Verification items for the finished model (mm, model axes). Give positions to 0.01 mm unless a question says otherwise; leave off trailing zeros. Order: outer loops, then holes, each group sorted by start corner. A loop starts at its lowest first (then second) coordinate and runs counter-clockwise, first axis right, second up. Notation, with made-up numbers: (33.25, -28.75) - (89.25, -28.75) arc R36 ccw to (89.25, 6.25) - close; hole circle Ø3 at (17.5, 56.25). An arc over 180 degrees is marked (long way). Answer as a JSON object with one key per item and string values.
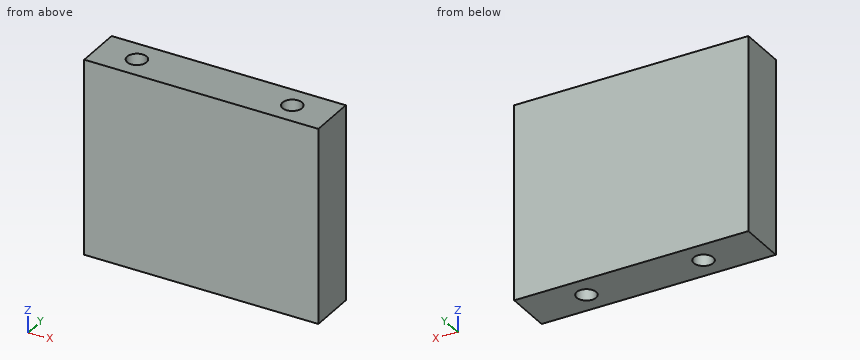
```python
from build123d import *

# Parameters (mm, degrees)
ESQUISSE1_W                                   = 30
ESQUISSE1_H                                   = 25
BOSS_EXTRU_1_DEPTH                            = 6
TROU_POUR_TARAUDAGE_POUR_TROU_TARAUD_M3_D     = 2.5
TROU_POUR_TARAUDAGE_POUR_TROU_TARAUD_M3_DEPTH = 10
TROU_POUR_TARAUDAGE_POUR_TROU_TARAUD_M3_TIP   = 0.751075774
TROU_POUR_TARAUDAGE_POUR_TROU_TARAUD_2_D      = 2.5
TROU_POUR_TARAUDAGE_POUR_TROU_TARAUD_2_DEPTH  = 11
TROU_POUR_TARAUDAGE_POUR_TROU_TARAUD_2_TIP    = 0.751075774


with BuildPart() as part:
    # Esquisse1 → Boss.-Extru.1 (new body)
    with BuildSketch(Plane(origin=(0, 0, 0), x_dir=(1, 0, 0), z_dir=(0, 1, 0))):
        Rectangle(ESQUISSE1_W, ESQUISSE1_H)
    extrude(amount=BOSS_EXTRU_1_DEPTH)

    # Trou pour taraudage pour trou taraud_ M3
    with Locations(Plane.XY.offset(12.5)):
        with Locations((-10, 3), (9.903892631, 3.003728502)):
            Hole(TROU_POUR_TARAUDAGE_POUR_TROU_TARAUD_M3_D / 2, depth=TROU_POUR_TARAUDAGE_POUR_TROU_TARAUD_M3_DEPTH)
            with Locations((0, 0, -(TROU_POUR_TARAUDAGE_POUR_TROU_TARAUD_M3_DEPTH + TROU_POUR_TARAUDAGE_POUR_TROU_TARAUD_M3_TIP / 2))):  # 118° drill point
                Cone(0, TROU_POUR_TARAUDAGE_POUR_TROU_TARAUD_M3_D / 2, TROU_POUR_TARAUDAGE_POUR_TROU_TARAUD_M3_TIP, mode=Mode.SUBTRACT)

    # Trou pour taraudage pour trou taraud 2
    with Locations(Plane(origin=(0, 0, -12.5), x_dir=(-1, 0, 0), z_dir=(0, 0, -1))):
        with Locations((-7.5, 3), (7.5, 3)):
            Hole(TROU_POUR_TARAUDAGE_POUR_TROU_TARAUD_2_D / 2, depth=TROU_POUR_TARAUDAGE_POUR_TROU_TARAUD_2_DEPTH)
            with Locations((0, 0, -(TROU_POUR_TARAUDAGE_POUR_TROU_TARAUD_2_DEPTH + TROU_POUR_TARAUDAGE_POUR_TROU_TARAUD_2_TIP / 2))):  # 118° drill point
                Cone(0, TROU_POUR_TARAUDAGE_POUR_TROU_TARAUD_2_D / 2, TROU_POUR_TARAUDAGE_POUR_TROU_TARAUD_2_TIP, mode=Mode.SUBTRACT)


solid = part.part
```
(1) Gauge pin test, flat ends, axial feed: pin 1 Ø8 at (x, z) = (-7, 9) entering from -Y; pin 2 Ø1.5 at (x, y) = (9.9, 3) entering from +Z. Record the tip position at first contact, or that the pin passes through.
Computed values:
{"pin 1": "stops at y = 0", "pin 2": "stops at z = 2.2"}
(2) Material ranges on line 1 along X through (y, z) = (3, -5); line 2 along Y through (x, z) = (-7.5, -5.75); line 3 along X through (y, z) = (3.65, 9.25), recorded low to high. Write a range as [from, to].
Computed values:
{"line 1": "x = [-15, -8.75], [-6.25, 6.25], [8.75, 15]", "line 2": "y = [0, 1.75], [4.25, 6]", "line 3": "x = [-15, -11.07], [-8.93, 8.83], [10.97, 15]"}
(3) Section check A-A (z = 3.75). Record the cut outline in (x, y).
Computed values:
{"outline": "(-15, 0) - (15, 0) - (15, 6) - (-15, 6) - close; hole circle Ø2.5 at (-10, 3); hole circle Ø2.5 at (9.9, 3)"}
